Here's how the part is built. I have some questions about the finished solid (model axes, mm). A direction names the side the tool comes from. Round coordinates to 2 decimals unless told otherwise and drop trailing zeros. Write each loop counter-clockwise with the first axis right and the second up, starting at its lowest first coordinate (ties: lowest second). Pieces come first, ordered by that corner, then holes. Notation, with made-up numbers: M 36,60 L 50,60 A31 cw 50,94 Z; hole C -19,78 d8. An arc over 180 degrees is marked long. Write item = value, one per line. Start each with the question number.
(1) I want a section at D-D (z = 15.5). List the corners of the cut face in (x, y) for me.
(2) I want a section at A-A (z = 34). List the corners of the cut face in (x, y) for me.
(3) If we mould it in two halves opening along X, with no side actions, what happens to faces 1 (the flat face through (-70, 14, 35)), 2 (the flat face through (-1, -2, 0)), 3 (the flat face through (75, -3, 25)), 4 (the flat face through (-75, -3, 25))? For each: released by +X, released by -X, zero draft, split by the parting line, or undercut.
(4) I need wall thicknesses on line 1 along Y through (x, z) = (-3, 23); line 2 along X through (y, z) = (-14.5, 17); line 3 along Y through (x, z) = (13.5, 16.5). Which ranges of each line are inside material? Lowest first, please.
(5) I want a section at C-C (x = 39). List the corners of the cut face in (y, z) for me.
(6) Will this pin go through, and if not, where does the flat tip stop? pin 1 Ø4 at (x, y) = (11, -27.5) entering from +Z.
(7) On a 3-axis mill with a long thin cutter (end or side, diameter ignored), from which of +Z, -Z, +X, -X, +Y, -Y can I reach the whole of each face in a straight line? I mean faces 5 (the flat face through (-1, -35, 25)), 6 (the flat face through (-1, 25, 35)). Say none if no direction works.
(8) I want a section at B-B (y = 5). List the corners of the cut face in (x, z) for me.
```python
from build123d import *

# Parameters (mm, degrees)
F0_W     = 150
F0_H     = 65
F0_W_2   = 67.5
F0_H_2   = 27.5
F0_W_3   = 140
F0_H_3   = 22.5
F1_DEPTH = 50
F2_DEPTH = 20
F3_DEPTH = 10


with BuildPart() as f1:
    # F0 (on Top) → F1 (new body)
    with BuildSketch(Plane.XY):
        with Locations((0, -2.5)):
            Rectangle(F0_W, F0_H)
        with Locations((-36.25, -16.25)):
            Rectangle(F0_W_2, F0_H_2, mode=Mode.SUBTRACT)
        with Locations((36.25, -16.25)):
            Rectangle(F0_W_2, F0_H_2, mode=Mode.SUBTRACT)
        with Locations((0, 13.75)):
            Rectangle(F0_W_3, F0_H_3, mode=Mode.SUBTRACT)
    extrude(amount=F1_DEPTH)

    # F0 (on Top) → F2 (join)
    with BuildSketch(Plane.XY):
        with Locations((0, 13.75)):
            Rectangle(F0_W_3, F0_H_3)
    extrude(amount=F2_DEPTH)

    # F0 (on Top) → F3 (join)
    with BuildSketch(Plane.XY):
        with Locations((-36.25, -16.25)):
            Rectangle(F0_W_2, F0_H_2)
        with Locations((36.25, -16.25)):
            Rectangle(F0_W_2, F0_H_2)
    extrude(amount=F3_DEPTH)


solid = f1.part
```
Returned:
q1.outline = M -75,-35 L 75,-35 L 75,30 L -75,30 Z; hole M -70,-30 L -2.5,-30 L -2.5,-2.5 L -70,-2.5 Z; hole M 2.5,-30 L 70,-30 L 70,-2.5 L 2.5,-2.5 Z
q2.outline = M -75,-35 L 75,-35 L 75,30 L -75,30 Z; hole M -70,-30 L -2.5,-30 L -2.5,-2.5 L -70,-2.5 Z; hole M -70,2.5 L 70,2.5 L 70,25 L -70,25 Z; hole M 2.5,-30 L 70,-30 L 70,-2.5 L 2.5,-2.5 Z
q3.face_1 = undercut
q3.face_2 = zero draft
q3.face_3 = released by +X
q3.face_4 = released by -X
q4.line_1 = -35 to -30, -2.5 to 2.5, 25 to 30
q4.line_2 = -75 to -70, -2.5 to 2.5, 70 to 75
q4.line_3 = -35 to -30, -2.5 to 30
q5.outline = M -35,0 L 30,0 L 30,50 L 25,50 L 25,20 L 2.5,20 L 2.5,50 L -2.5,50 L -2.5,10 L -30,10 L -30,50 L -35,50 Z
q6.pin_1 = 10
q7.face_5 = +Z, -Z, +X, -X, -Y
q7.face_6 = +Z
q8.outline = M -75,0 L 75,0 L 75,50 L 70,50 L 70,20 L -70,20 L -70,50 L -75,50 Z
